from build123d import *


with BuildPart() as part:
    # Sketch1 → Revolve1 (revolve)
    with BuildSketch(Plane.XY):
        with BuildLine():
            Line((0.3, 4), (6.7, 4))
            ThreePointArc((6.7, 4), (6.912132034, 4.087867966), (7, 4.3))
            Line((7, 4.3), (7, 6.1))
            Line((7, 6.1), (6.4, 6.1))
            Line((6.4, 6.1), (6.4, 9.65))
            Line((6.4, 9.65), (7, 9.65))
            Line((7, 9.65), (7, 10.7))
            ThreePointArc((7, 10.7), (6.912132034, 10.912132034), (6.7, 11))
            Line((6.7, 11), (0.3, 11))
            ThreePointArc((0.3, 11), (0.087867966, 10.912132034), (0, 10.7))
            Line((0, 10.7), (0, 9.65))
            Line((0, 9.65), (0.6, 9.65))
            Line((0.6, 9.65), (0.6, 6.1))
            Line((0.6, 6.1), (0, 6.1))
            Line((0, 6.1), (0, 4.3))
            ThreePointArc((0, 4.3), (0.087867966, 4.087867966), (0.3, 4))
        make_face()
    revolve(axis=Axis((-0.002803158, 0, 0), (1, 0, 0)))


solid = part.part
Geometry check sheet. Reference: the model listing, model coordinates, mm. A direction names the side the tool comes from. Give positions to 0.01 mm unless a question says otherwise; leave off trailing zeros. Order: outer loops, then holes, each group sorted by start corner. A loop starts at its lowest first (then second) coordinate and runs counter-clockwise, first axis right, second up. Notation, with made-up numbers: M 22,34 L 35,34 A11 cw 35,43 Z; hole C 73.5,80 d5. An arc over 180 degrees is marked long. Use a Markdown table: item, result.
Item 1: Material ranges on line 1 along Z through (x, y) = (0.4, 0); line 2 along Y through (x, z) = (6.5, 2.5); line 3 along X through (y, z) = (7.75, -4.25), recorded low to high.
Answers follow:
| item | result |
|---|---|
| line 1 | z = -11 to -9.65, -6.1 to -4, 4 to 6.1, 9.65 to 11 |
| line 2 | y = -10.71 to -9.32, -5.56 to -3.12, 3.12 to 5.56, 9.32 to 10.71 |
| line 3 | x = 0.6 to 6.4 |
Item 2: Section check C-C (x = 4.5). Record the cut outline in (y, z), and give its area (3 significant figures).
Answers follow:
| item | result |
|---|---|
| outline | C 0,0 d22; hole C 0,0 d8 |
| area | 330 mm2 |
Item 3: Depth check by flat-ended pin: P1, Ø1, axis at y = 7.5, z = -5, coming from the +X side; P2, Ø7, axis at y = 0, z = 0, coming from the -X side; P3, Ø3, axis at x = 3.5, z = 4, coming from the -Y side. Enter the tip coordinate at first touch or a pass-through.
Answers follow:
| item | result |
|---|---|
| P1 | stops at x = 6.4 |
| P2 | passes through |
| P3 | stops at y = -10.71 |
Item 4: Draft check along Z on faces 4 (the cylindrical face through (3.46, -2.38, -10.74)), 5 (the cylindrical face through (0.296, -6.094, 0.268)), 6 (the flat face through (7, 2, 10)). Enter one of: +Z half, -Z half, draft (parallel to the pull), parting line (faces both ways), or undercut.
Answers follow:
| item | result |
|---|---|
| face 4 | parting line |
| face 5 | undercut |
| face 6 | draft |
Item 5: Tool access check on faces 1 (the flat face through (0, -2, 10)), 2 (the cylindrical face through (0.304, 9.204, 2.899)), 3 (the cylindrical face through (6.704, 9.204, 2.899)). Record the directions out of +Z, -Z, +X, -X, +Y, -Y that give a thin tool (end or side, any length) a straight path to the whole face; none if there is none.
Answers follow:
| item | result |
|---|---|
| face 1 | +Z, -Z, -X, +Y, -Y |
| face 2 | -X |
| face 3 | +X |
